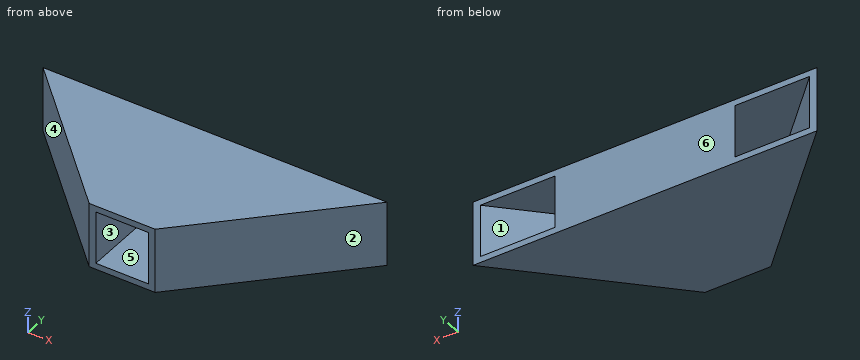
```python
from build123d import *

# Parameters (mm, degrees)
F1_DEPTH = 16
F3_START = -1.5
F3_DEPTH = 13
F4_SIZE  = 11.5
F5_W     = 13
F5_H     = 13
F6_DEPTH = 32


with BuildPart() as f1:
    # F0 (on Top) → F1 (new body)
    with BuildSketch(Plane.XY):
        Polygon((-42.4264068712, 42.4264068712), (0, 0), (42.4264068712, 42.4264068712), align=None)
    extrude(amount=F1_DEPTH)

    # F2 (on face) → F3 (cut)
    with BuildSketch(Plane.XY.offset(16).offset(F3_START)):
        Polygon((-51.2700945749, 53.0700945749), (-15.5563491861, 17.3563491861), (-6.3639610307, 26.5487373415), (-42.0777064195, 62.2624827303), align=None)
        Polygon((6.3639610307, 26.5487373415), (15.5563491861, 17.3563491861), (49.0367116487, 50.8367116487), (39.8443234933, 60.0290998041), align=None)
    extrude(amount=-F3_DEPTH, mode=Mode.SUBTRACT)

    # F4
    f4_edges = [f1.edges().sort_by_distance(p)[0] for p in [
        (0, 0, 8),
    ]]
    chamfer(f4_edges, length=F4_SIZE)

    # F5 (on face) → F6 (cut)
    with BuildSketch(Plane.XZ.offset(-8.1317279836)):
        with Locations((0, 8)):
            Rectangle(F5_W, F5_H)
    extrude(amount=-F6_DEPTH, mode=Mode.SUBTRACT)


solid = f1.part
```
Part model, mm, in its own coordinate system. Face numbers are marked on the shaded views. A direction names the side the tool comes from. Round coordinates to 2 decimals unless told otherwise and drop trailing zeros. Write each loop counter-clockwise with the first axis right and the second up, starting at its lowest first coordinate (ties: lowest second). Pieces come first, ordered by that corner, then holes. Notation, with made-up numbers: M -15.5,23.5 L 14.5,23.5 A16 cw 14.5,54.5 Z; hole C 81,33 d10. An arc over 180 degrees is marked long. One line per question, with ' | ' between items.
(1) Pin check, flat tips, straight feed: pin 1 (2 mm diameter, centred on x = -11, z = 12.5, fed in from -Y); pin 2 (4 mm diameter, centred on y = 13.5, z = 5.5, fed in from -X); pin 3 (4 mm diameter, centred on x = -13.5, z = 5.5, fed in from -Y). Stop position of each tip, or through.
Answer key:
pin 1: stops at y = 10 | pin 2: stops at x = -15.5 | pin 3: stops at y = 11.5
(2) Saw through at A-A on y = 11. Write the cut outline in (x, z), then the cut area to 3 significant figures.
Answer key:
outline: M -11,0 L 11,0 L 11,16 L -11,16 Z; hole M -6.5,1.5 L 6.5,1.5 L 6.5,14.5 L -6.5,14.5 Z | area: 183 mm^2
(3) Two-plate mould, pull along X, no slides. Class the marked faces 4, 5 and 6: released by +X, released by -X, zero draft, split by the parting line, or undercut.
Answer key:
face 4: released by -X | face 5: undercut | face 6: zero draft
(4) Saw through at D-D on y = 32. Write the cut outline in (x, z), then the cut area to 3 significant figures.
Answer key:
outline: M -32,0 L 32,0 L 32,16 L -32,16 Z; hole M -30.2,1.5 L -11.82,1.5 L -11.82,14.5 L -30.2,14.5 Z; hole M -6.5,1.5 L 6.5,1.5 L 6.5,14.5 L -6.5,14.5 Z; hole M 11.82,1.5 L 30.2,1.5 L 30.2,14.5 L 11.82,14.5 Z | area: 377 mm^2
(5) 3-axis set-ups, long thin cutter, end or side, ignore diameter. For the marked faces 1, 2 and 3: which of +Z, -Z, +X, -X, +Y, -Y reach the whole face in a straight line?
Answer key:
face 1: none | face 2: +Z, -Z, +X, -Y | face 3: -Y
(6) Saw through at B-B on z = 7.75. Write the cut outline in (x, y), then the cut area to 3 significant figures.
Answer key:
outline: M -42.43,42.43 L -8.13,8.13 L -6.5,8.13 L -6.5,26.41 L -15.56,17.36 L -40.63,42.43 Z; M -22.24,42.43 L -6.5,26.68 L -6.5,40.13 L 6.5,40.13 L 6.5,26.68 L 22.24,42.43 Z; M 6.5,8.13 L 8.13,8.13 L 42.43,42.43 L 40.63,42.43 L 15.56,17.36 L 6.5,26.41 Z | area: 565 mm^2
(7) Saw through at C-C on x = -34. Write the cut outline in (y, z), then the cut area to 3 significant figures.
Answer key:
outline: M 34,0 L 42.43,0 L 42.43,1.5 L 35.8,1.5 L 35.8,14.5 L 42.43,14.5 L 42.43,16 L 34,16 Z | area: 48.7 mm^2
(8) Probe line 1 along Z through (x, y) = (-25, 28); line 2 along X through (y, z) = (28.5, 14); line 3 along X through (y, z) = (32, 9.25). List the from-to ranges inside material, lowest first.
Answer key:
line 1: z = 0 to 1.5, 14.5 to 16 | line 2: x = -28.5 to -26.7, -8.32 to -6.5, 6.5 to 8.32, 26.7 to 28.5 | line 3: x = -32 to -30.2, -11.82 to -6.5, 6.5 to 11.82, 30.2 to 32
